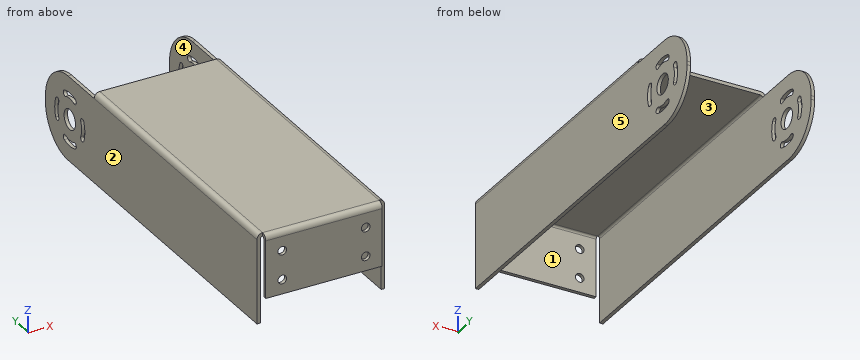
```python
from build123d import *

# Parameters (mm, degrees)
SKETCH_1_W                  = 40.5
SKETCH_1_H                  = 100
SM_BASE_FLANGE_1_DEPTH      = 1.2
SM_EDGE_FLANGE_1_DEPTH      = 100
SM_EDGE_FLANGE_1_BEND_DEPTH = 100
SM_EDGE_FLANGE_3_DEPTH      = 40.5
SKETCH_25_R                 = 1.5
CUT_EXTRUDE_1_DEPTH         = 10
SKETCH_26_W                 = 1.2
SKETCH_26_H                 = 29.2634
EXTRUDE_1_DEPTH             = 30
SKETCH_29_R                 = 3.5
CUT_EXTRUDE_2_DEPTH         = 87
FILLET_1_R                  = 14


# Sheet-metal steps are written as plain solids
with BuildPart() as part:
    # Sketch 1 → 基材-凸緣1 (new body)
    with BuildSketch(Plane.XY):
        with Locations((-29.069965263, -8.639189189)):
            Rectangle(SKETCH_1_W, SKETCH_1_H)
    extrude(amount=-SM_BASE_FLANGE_1_DEPTH)

    # 邊線-凸緣1 section (across the edge) → 邊線-凸緣1 (add)
    with BuildSketch(Plane(origin=(-8.083365263, 41.360810811, -1.2), x_dir=(-1, 0, 0), z_dir=(0, -1, 0))):
        with BuildLine():
            Line((-1.2, 0.7366), (-1.2, 30))
            Line((-1.2, 30), (0, 30))
            Line((0, 30), (0, 0.7366))
            ThreePointArc((0, 0.7366), (0.215745145, 0.215745145), (0.7366, 0))
            Line((0.7366, 0), (0.7366, -1.2))
            ThreePointArc((0.7366, -1.2), (-0.632782992, -0.632782992), (-1.2, 0.7366))
        make_face()
    extrude(amount=SM_EDGE_FLANGE_1_DEPTH)

    # 邊線-凸緣1 section 2 (across the edge) → 邊線-凸緣1 bend (add)
    with BuildSketch(Plane(origin=(-50.056565263, -58.639189189, -1.2), x_dir=(1, 0, 0), z_dir=(0, 1, 0))):
        with BuildLine():
            Line((-1.2, 0.7366), (-1.2, 30))
            Line((-1.2, 30), (0, 30))
            Line((0, 30), (0, 0.7366))
            ThreePointArc((0, 0.7366), (0.215745145, 0.215745145), (0.7366, 0))
            Line((0.7366, 0), (0.7366, -1.2))
            ThreePointArc((0.7366, -1.2), (-0.632782992, -0.632782992), (-1.2, 0.7366))
        make_face()
    extrude(amount=SM_EDGE_FLANGE_1_BEND_DEPTH)

    # 邊線-凸緣3 section (across the edge) → 邊線-凸緣3 (add)
    with BuildSketch(Plane(origin=(-8.819965263, -59.375789189, -1.2), x_dir=(0, 1, 0), z_dir=(-1, 0, 0))):
        with BuildLine():
            Line((-1.2, 0.7366), (-1.2, 20.735))
            Line((-1.2, 20.735), (0, 20.735))
            Line((0, 20.735), (0, 0.7366))
            ThreePointArc((0, 0.7366), (0.215745145, 0.215745145), (0.7366, 0))
            Line((0.7366, 0), (0.7366, -1.2))
            ThreePointArc((0.7366, -1.2), (-0.632782992, -0.632782992), (-1.2, 0.7366))
        make_face()
    extrude(amount=SM_EDGE_FLANGE_3_DEPTH)

    # 草圖25 → 除料-伸長1 (cut)
    with BuildSketch(Plane.XZ.offset(60.575789189)):
        with Locations(Location((-43.579965263, -6.9366, 0), (0, 0, 270))):
            Circle(SKETCH_25_R)
        with Locations(Location((-43.579965263, -16.935, 0), (0, 0, 90))):
            Circle(SKETCH_25_R)
        with Locations(Location((-14.559965263, -16.935, 0), (0, 0, 270))):
            Circle(SKETCH_25_R)
        with Locations(Location((-14.559965263, -6.9366, 0), (0, 0, 90))):
            Circle(SKETCH_25_R)
    extrude(amount=-CUT_EXTRUDE_1_DEPTH, mode=Mode.SUBTRACT)

    # 草圖26 → 填料-伸長1 (add)
    with BuildSketch(Plane(origin=(0, 41.360810811, 0), x_dir=(1, 0, 0), z_dir=(0, 1, 0))):
        with Locations((-50.656565263, 16.5683)):
            Rectangle(SKETCH_26_W, SKETCH_26_H)
        with Locations((-7.483365263, 16.5683)):
            Rectangle(SKETCH_26_W, SKETCH_26_H)
    extrude(amount=EXTRUDE_1_DEPTH)

    # 草圖29 → 除料-伸長2 (cut)
    with BuildSketch(Plane(origin=(-6.883365263, 0, 0), x_dir=(0, 0, -1), z_dir=(1, 0, 0))):
        with Locations((16.5683, 56.360810811)):
            Circle(SKETCH_29_R)
        with BuildLine():
            ThreePointArc((25.185054053, 52.997174447), (25.8183, 56.360810811), (25.185054053, 59.724447174))
            ThreePointArc((25.185054053, 59.724447174), (23.889876711, 60.29235179), (23.321972096, 58.997174447))
            ThreePointArc((23.321972096, 58.997174447), (23.8183, 56.360810811), (23.321972096, 53.724447174))
            ThreePointArc((23.321972096, 53.724447174), (23.889876711, 52.429269832), (25.185054053, 52.997174447))
        make_face()
        with BuildLine():
            ThreePointArc((13.204663636, 64.977564864), (12.636759021, 63.682387522), (13.931936364, 63.114482907))
            ThreePointArc((13.931936364, 63.114482907), (16.5683, 63.610810811), (19.204663636, 63.114482907))
            ThreePointArc((19.204663636, 63.114482907), (20.499840979, 63.682387522), (19.931936364, 64.977564864))
            ThreePointArc((19.931936364, 64.977564864), (16.5683, 65.610810811), (13.204663636, 64.977564864))
        make_face()
        with BuildLine():
            ThreePointArc((13.204663636, 47.744056758), (16.5683, 47.110810811), (19.931936364, 47.744056758))
            ThreePointArc((19.931936364, 47.744056758), (20.499840979, 49.0392341), (19.204663636, 49.607138715))
            ThreePointArc((19.204663636, 49.607138715), (16.5683, 49.110810811), (13.931936364, 49.607138715))
            ThreePointArc((13.931936364, 49.607138715), (12.636759021, 49.0392341), (13.204663636, 47.744056758))
        make_face()
        with BuildLine():
            ThreePointArc((7.951545947, 59.724447174), (7.3183, 56.360810811), (7.951545947, 52.997174447))
            ThreePointArc((7.951545947, 52.997174447), (9.246723289, 52.429269832), (9.814627904, 53.724447174))
            ThreePointArc((9.814627904, 53.724447174), (9.3183, 56.360810811), (9.814627904, 58.997174447))
            ThreePointArc((9.814627904, 58.997174447), (9.246723289, 60.29235179), (7.951545947, 59.724447174))
        make_face()
    extrude(amount=-CUT_EXTRUDE_2_DEPTH, mode=Mode.SUBTRACT)

    # 圓角1
    fillet_1_edges = [part.edges().sort_by_distance(p)[0] for p in [
        (-50.656565263, 71.360810811, -31.2),
        (-50.656565263, 71.360810811, -1.9366),
        (-7.483365263, 71.360810811, -31.2),
        (-7.483365263, 71.360810811, -1.9366),
    ]]
    fillet(fillet_1_edges, radius=FILLET_1_R)


solid = part.part
```
Work out the finished part from the listing and answer in its coordinate system (mm). Face numbers are marked on the shaded views. A direction names the side the tool comes from. Give positions to 0.01 mm unless a question says otherwise; leave off trailing zeros. Write each loop counter-clockwise with the first axis right and the second up, starting at its lowest first coordinate (ties: lowest second). Pieces come first, ordered by that corner, then holes.
(1) Flat-ended cylindrical pins translate along their axes: pin 1 Ø0.6 at (x, y) = (-8, 50) entering from +Z; pin 2 Ø1.5 at (y, z) = (-59.5, -6) entering from -X; pin 3 Ø5 at (x, y) = (-28.5, 42.5) entering from -Z; pin 4 Ø1.5 at (x, z) = (-50, -16) entering from -Y. Find the tip coordinate at first contact, or state that the pin passes through.
Final values:
pin 1: stops at z = -1.94
pin 2: stops at x = -49.32
pin 3: stops at z = -1.2
pin 4: stops at y = -60.58
(2) The mould has two halves that part along X. Classify the marked faces 1, 2 and 3: pulls with the +X half, pulls with the -X half, needs draft (parallel to the pull), parting line crosses it, or undercut.
Final values:
face 1: needs draft
face 2: pulls with the -X half
face 3: undercut
(3) The part is cut by section B-B on x = -33.5. Write down the section's boundary in (y, z) (3 decimals).
Final values:
outline: (-60.576, -21.935) - (-59.376, -21.935) - (-59.376, -1.937) arc R0.737 cw to (-58.639, -1.2) - (41.361, -1.2) - (41.361, 0) - (-58.639, 0) arc R1.937 ccw to (-60.576, -1.937) - close
(4) The part is cut by section A-A on z = -28.5. Write down the section's boundary in (x, y), plus the area to 3 significant figures.
Final values:
outline: (-51.26, -58.64) - (-50.06, -58.64) - (-50.06, 65.63) - (-51.26, 65.63) - close; (-8.08, -58.64) - (-6.88, -58.64) - (-6.88, 65.63) - (-8.08, 65.63) - close
area: 298 mm2
(5) Which of the six approach directions +Z, -Z, +X, -X, +Y, -Y give full straight-line access (tool end or side, diameter ignored) to the marked faces 4 and 5?
Final values:
face 4: -Z, +Y, -Y
face 5: +Z, -Z, +X, +Y, -Y
(6) Straight lines are drawn through the part: line 1 (X direction, y = 60, z = -4.5); line 2 (Y direction, x = -35, z = -5.5); line 3 (Z direction, x = -23, y = 36). For each, find the intervals that lie inside material, in ascending order.
Final values:
line 1: x = -51.26 to -50.06, -8.08 to -6.88
line 2: y = -60.58 to -59.38
line 3: z = -1.2 to 0
(7) The part is cut by section C-C on y = -24. Write down the section's boundary in (x, z), plus the area to 3 significant figures.
Final values:
outline: (-51.26, -31.2) - (-50.06, -31.2) - (-50.06, -1.94) arc R0.74 cw to (-49.32, -1.2) - (-8.82, -1.2) arc R0.74 cw to (-8.08, -1.94) - (-8.08, -31.2) - (-6.88, -31.2) - (-6.88, -1.94) arc R1.94 ccw to (-8.82, 0) - (-49.32, 0) arc R1.94 ccw to (-51.26, -1.94) - close
area: 124 mm2
